from build123d import *

# Parameters (mm, degrees)
CUT_EXTRUDE1_DEPTH          = 19.304
F_1_4_28_TAPPED_HOLE1_D     = 5.4102
F_1_4_28_TAPPED_HOLE1_DEPTH = 6.096


with BuildPart() as part:
    # Sketch1 → Revolve1 (revolve)
    with BuildSketch(Plane.XY):
        with BuildLine():
            Line((0, 0), (0, 15.875))
            Line((0, 15.875), (6.35, 15.875))
            Line((6.35, 15.875), (6.35, 12.7))
            ThreePointArc((6.35, 12.7), (7.27993597, 10.45493597), (9.525, 9.525))
            Line((9.525, 9.525), (20.955, 9.525))
            ThreePointArc((20.955, 9.525), (23.20006403, 8.59506403), (24.13, 6.35))
            Line((24.13, 6.35), (24.13, 0))
            Line((24.13, 0), (0, 0))
        make_face()
    revolve(axis=Axis((24.13, 0, 0), (-1, 0, 0)))

    # Sketch2 → Cut-Extrude1 (cut)
    with BuildSketch(Plane.ZY):
        with BuildLine():
            Line((-3.485565844, 3.429), (3.485565844, 3.429))
            ThreePointArc((3.485565844, 3.429), (0, -4.8895), (-3.485565844, 3.429))
        make_face()
    extrude(amount=-CUT_EXTRUDE1_DEPTH, mode=Mode.SUBTRACT)

    # 1/4-28 Tapped Hole1
    with Locations(Plane(origin=(0, 9.525, 0), x_dir=(1, 0, 0), z_dir=(0, 1, 0))):
        with Locations((13.97, 0)):
            Hole(F_1_4_28_TAPPED_HOLE1_D / 2, depth=F_1_4_28_TAPPED_HOLE1_DEPTH)


solid = part.part
Read the model definition and answer for the solid it produces. Units are mm, in the model's axes. A direction names the side the tool comes from. Coordinates: 2 decimals unless noted, no trailing zeros. Return JSON: item names as keys, results as strings.
(1) Consider line 1 along Y through (x, z) = (6.25, 0) (1 decimal); line 2 along Z through (x, y) = (1.5, 0) (1 decimal); line 3 along X through (y, z) = (12.5, 8). Determine where each line is inside the solid, lowest interval first. Write a range as from..to.
Answers below:
{"line 1": "-15.9..-4.9, 3.4..15.9", "line 2": "-15.9..-4.9, 4.9..15.9", "line 3": "0..6.35"}
(2) Which of the six approach directions +Z, -Z, +X, -X, +Y, -Y give full straight-line access (tool end or side, diameter ignored) to faces 1 (the cylindrical face through (12.72, 6.43, 2.4)), 2 (the cylindrical face through (9.517, -4.887, 0.161)), 3 (the flat face through (6.35, -7, -11))?
Answers below:
{"face 1": "+Y", "face 2": "-X", "face 3": "+X"}
(3) For a pull along Y with two mould halves and no side action, classify faces 4 (the flat face through (19.304, -1, 0)), 5 (the flat face through (0, 4, 0)), 6 (the cylindrical face through (15.32, -7.559, 5.796)) as pulls with the +Y half, pulls with the -Y half, needs draft (parallel to the pull), parting line crosses it, or undercut.
Answers below:
{"face 4": "undercut", "face 5": "needs draft", "face 6": "parting line crosses it"}
(4) Each of these flat-tipped pins is pushed along its axis until it touches: P1, Ø8, axis at x = 21, z = 7, coming from the -Y side; P2, Ø2.5, axis at y = -2.5, z = 2, coming from the -X side; P3, Ø5.5, axis at x = 14, z = 0, coming from the -Y side (3 decimals). Where does it stop, or does it pass through?
Answers below:
{"P1": "y = -9.04", "P2": "x = 19.3", "P3": "y = -9.525"}
